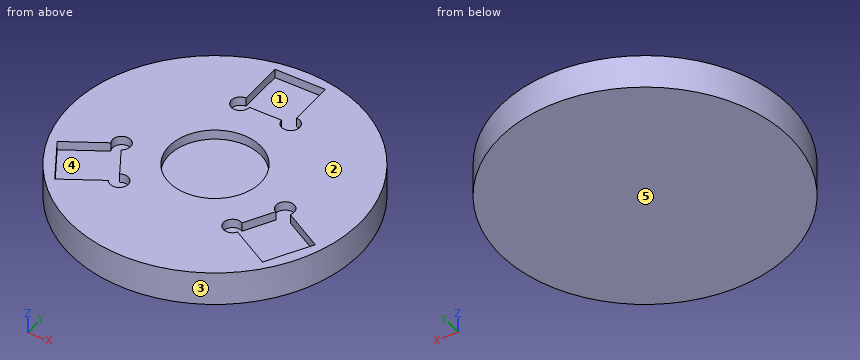
from build123d import *

# Parameters (mm, degrees)
SKETCH1_R           = 50.8
BOSS_EXTRUDE1_DEPTH = 11.9888
SKETCH3_W           = 17.57426
SKETCH3_H           = 19.05
POCKET_DEPTH        = 3.175
SKETCH7_R           = 3.175
CORNER_RELIEF_DEPTH = 3.175
CIRPATTERN1_COUNT   = 3
SKETCH5_R           = 16.002
MAGNET_INSET_DEPTH  = 3.429


with BuildPart() as part:
    # Sketch1 → Boss-Extrude1 (new body)
    with BuildSketch(Plane.XY):
        with Locations(Location((0, 0, 0), (0, 0, 180))):
            Circle(SKETCH1_R)
    extrude(amount=BOSS_EXTRUDE1_DEPTH)

    # Sketch3 → pocket (cut)
    with BuildSketch(Plane.XY.offset(11.9888)):
        with Locations((0, 37.465)):
            Rectangle(SKETCH3_W, SKETCH3_H)
    pocket = extrude(amount=-POCKET_DEPTH, mode=Mode.SUBTRACT)

    # Sketch7 → corner relief (cut)
    with BuildSketch(Plane.XY.offset(11.9888)):
        with Locations((-8.78713, 27.94)):
            Circle(SKETCH7_R)
        with Locations((8.78713, 27.94)):
            Circle(SKETCH7_R)
    corner_relief = extrude(amount=-CORNER_RELIEF_DEPTH, mode=Mode.SUBTRACT)

    # CirPattern1: pocket, corner relief ×3 about axis
    cirpattern1_axis = Axis((0, 0, 0), (0, 0, 1))
    add([pocket.rotate(cirpattern1_axis, i * 360 / CIRPATTERN1_COUNT) for i in range(1, CIRPATTERN1_COUNT)], mode=Mode.SUBTRACT)
    add([corner_relief.rotate(cirpattern1_axis, i * 360 / CIRPATTERN1_COUNT) for i in range(1, CIRPATTERN1_COUNT)], mode=Mode.SUBTRACT)

    # Sketch5 → magnet inset (cut)
    with BuildSketch(Plane.XY.offset(11.9888)):
        Circle(SKETCH5_R)
    extrude(amount=-MAGNET_INSET_DEPTH, mode=Mode.SUBTRACT)


solid = part.part
Verification items for the finished model (mm, model axes). Face numbers are marked on the shaded views. A direction names the side the tool comes from. Coordinates: 2 decimals unless noted, no trailing zeros. Order: outer loops, then holes, each group sorted by start corner. A loop starts at its lowest first (then second) coordinate and runs counter-clockwise, first axis right, second up. Notation, with made-up numbers: (-19, 17) -> (21, 17) arc R12 cw to (21, 30) -> close; hole circle Ø2 at (1.5, 5). An arc over 180 degrees is marked (long way). Use CSV: the item, a comma, the result in double quotes. Start each with the question number.
Q1. Section check C-C, the plane y = 0. Record the cut outline in (x, z), and give its area (3 significant figures).
Q2. Thickness scan on line 1 along Y through (x, z) = (-4.5, 11); line 2 along Y through (x, z) = (41.5, 9.5); line 3 along Z through (x, y) = (-11.5, 1.5). Record the ranges inside material, lowest first.
Q3. Section check A-A, the plane x = 0. Record the cut outline in (y, z), and give its area (3 significant figures).
Q4. Section check B-B, the plane z = 10.5. Record the cut outline in (x, y) (3 decimals), and give its area (3 significant figures).
Q5. Depth check by flat-ended pin: P1, Ø3, axis at y = -2.5, z = 8.5, coming from the +X side; P2, Ø4, axis at y = -16.5, z = 2, coming from the -X side; P3, Ø1, axis at x = 0, z = 10, coming from the -Y side. Enter the tip coordinate at first touch or a pass-through.
Q6. Section check D-D, the plane z = 5. Record the cut outline in (x, y).
Q7. Tool access check on the marked faces 1 and 2. Record the directions out of +Z, -Z, +X, -X, +Y, -Y that give a thin tool (end or side, any length) a straight path to the whole face; none if there is none.
Q8. Draft check along X on the marked faces 3, 4 and 5. Enter one of: +X half, -X half, draft (parallel to the pull), parting line (faces both ways), or undercut.
Returned:
1,outline,"(-50.8, 0) -> (50.8, 0) -> (50.8, 11.99) -> (16, 11.99) -> (16, 8.56) -> (-16, 8.56) -> (-16, 11.99) -> (-50.8, 11.99) -> close"
1,area,"1,110 mm^2"
2,line 1,"y = -50.6 to -15.36, 15.36 to 27.94, 46.99 to 50.6"
2,line 2,"y = -29.3 to -22.1, -13.81 to 29.3"
2,line 3,"z = 0 to 8.56"
3,outline,"(-50.8, 0) -> (50.8, 0) -> (50.8, 11.99) -> (46.99, 11.99) -> (46.99, 8.81) -> (27.94, 8.81) -> (27.94, 11.99) -> (16, 11.99) -> (16, 8.56) -> (-16, 8.56) -> (-16, 11.99) -> (-50.8, 11.99) -> close"
3,area,"1,050 mm^2"
4,outline,"circle Ø101.6 at (0, 0); hole (-45.088, -15.885) -> (-36.301, -31.105) -> (-22.553, -23.167) arc R3.175 ccw (long way) to (-21.391, -18.83) -> (-27.003, -9.11) arc R3.175 ccw (long way) to (-31.34, -7.948) -> close; hole circle Ø32.004 at (0, 0); hole (-8.787, 31.115) arc R3.175 ccw (long way) to (-5.612, 27.94) -> (5.612, 27.94) arc R3.175 ccw (long way) to (8.787, 31.115) -> (8.787, 46.99) -> (-8.787, 46.99) -> close; hole (21.391, -18.83) arc R3.175 ccw (long way) to (22.553, -23.167) -> (36.301, -31.105) -> (45.088, -15.885) -> (31.34, -7.948) arc R3.175 ccw (long way) to (27.003, -9.11) -> close"
4,area,"6,160 mm^2"
5,P1,"stops at x = 50.79"
5,P2,"stops at x = -48.69"
5,P3,"stops at y = -50.8"
6,outline,"circle Ø101.6 at (0, 0)"
7,face 1,"+Z"
7,face 2,"+Z, +X, -X, +Y, -Y"
8,face 3,"parting line"
8,face 4,"undercut"
8,face 5,"draft"
